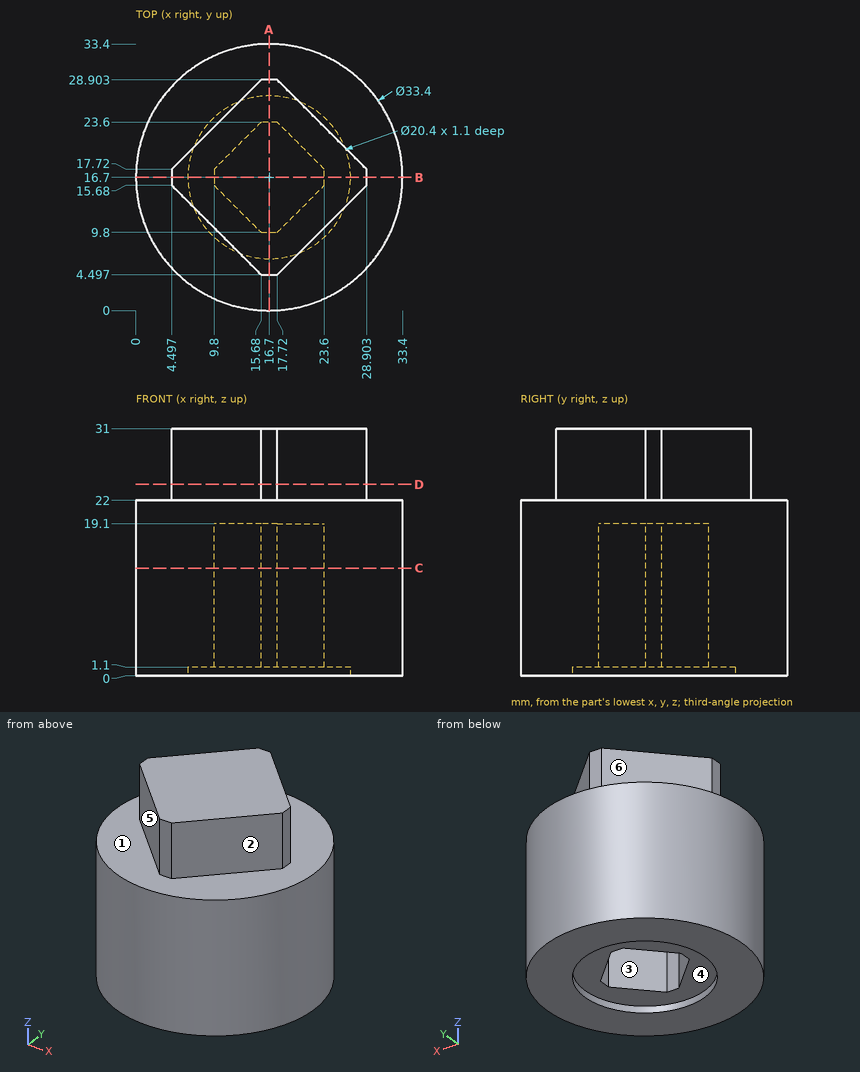
Job drawing, mm, ordinate dimensions from the low corner. One solid piece. A direction names the side the tool comes from. Give positions to 0.01 mm unless a question says otherwise; leave off trailing zeros. Loops run counter-clockwise (first coordinate to the right, second up) from the corner with the lowest first, then second, coordinate; pieces in that order, holes last. Notation, with made-up numbers: M -13.5,71.25 L 23.5,71.25 A29 cw 23.5,104.25 Z; hole C -1,70.25 d5. An arc over 180 degrees is marked long. Put each result on its own line as item: value. Start each with the question number.
1) Saw through at D-D (z = 24). List the corners of the cut face in (x, y).
2) 3-axis set-ups, long thin cutter, end or side, ignore diameter. For the marked faces 4, 5 and 6: which of +Z, -Z, +X, -X, +Y, -Y reach the whole face in a straight line?
3) Probe probe 1 along Y at (x, z) = (16.7, 0.4); probe 2 along Z at (x, y) = (8, 14); probe 3 along Z at (x, y) = (30, 8). List the from-to ranges inside material, lowest first.
4) Saw through at C-C (z = 13.5). List the corners of the cut face in (x, y).
5) Pull direction Y, two halves, no side cores. Call the marked faces 1, 2 and 3: +Y half, -Y half, draft (parallel to the pull), parting line (faces both ways), or undercut.
6) Saw through at A-A (x = 16.7). List the corners of the cut face in (y, z).
7) Flat gauge pins, fed straight in: pin 1 (6 mm diameter, centred on x = 21.5, y = 21.5, fed in from -Z); pin 2 (1.6 mm diameter, centred on y = 17, z = 28.5, fed in from -X); pin 3 (4 mm diameter, centred on x = 25, z = 28, fed in from -Y). Where does each tip first touch, or does it go through?
Numbers:
1. outline: M 4.5,15.68 L 15.68,4.5 L 17.72,4.5 L 28.9,15.68 L 28.9,17.72 L 17.72,28.9 L 15.68,28.9 L 4.5,17.72 Z
2. face 4: -Z
2. face 5: +Z, -X, -Y
2. face 6: +Z, -X, +Y
3. probe 1: 0 to 6.5, 26.9 to 33.4
3. probe 2: 1.1 to 31
3. probe 3: 0 to 22
4. outline: C 16.7,16.7 d33.4; hole M 9.8,15.68 L 15.68,9.8 L 17.72,9.8 L 23.6,15.68 L 23.6,17.72 L 17.72,23.6 L 15.68,23.6 L 9.8,17.72 Z
5. face 1: draft
5. face 2: -Y half
5. face 3: undercut
6. outline: M 0,0 L 6.5,0 L 6.5,1.1 L 9.8,1.1 L 9.8,19.1 L 23.6,19.1 L 23.6,1.1 L 26.9,1.1 L 26.9,0 L 33.4,0 L 33.4,22 L 28.9,22 L 28.9,31 L 4.5,31 L 4.5,22 L 0,22 Z
7. pin 1: z = 1.1
7. pin 2: x = 4.5
7. pin 3: y = 9.78
